Study the drawing (mm; zero at the part's minimum x, y, z) and answer. A direction names the side the tool comes from. Coordinates: 2 decimals unless noted, no trailing zeros. Order: outer loops, then holes, each group sorted by start corner. A loop starts at its lowest first (then second) coordinate and runs counter-clockwise, first axis right, second up. Notation, with made-up numbers: M 82.25,1.25 L 128.25,1.25 A22 cw 128.25,25.25 Z; hole C 7,59 d1. An arc over 180 degrees is marked long. Put each result on its own line as item: value.
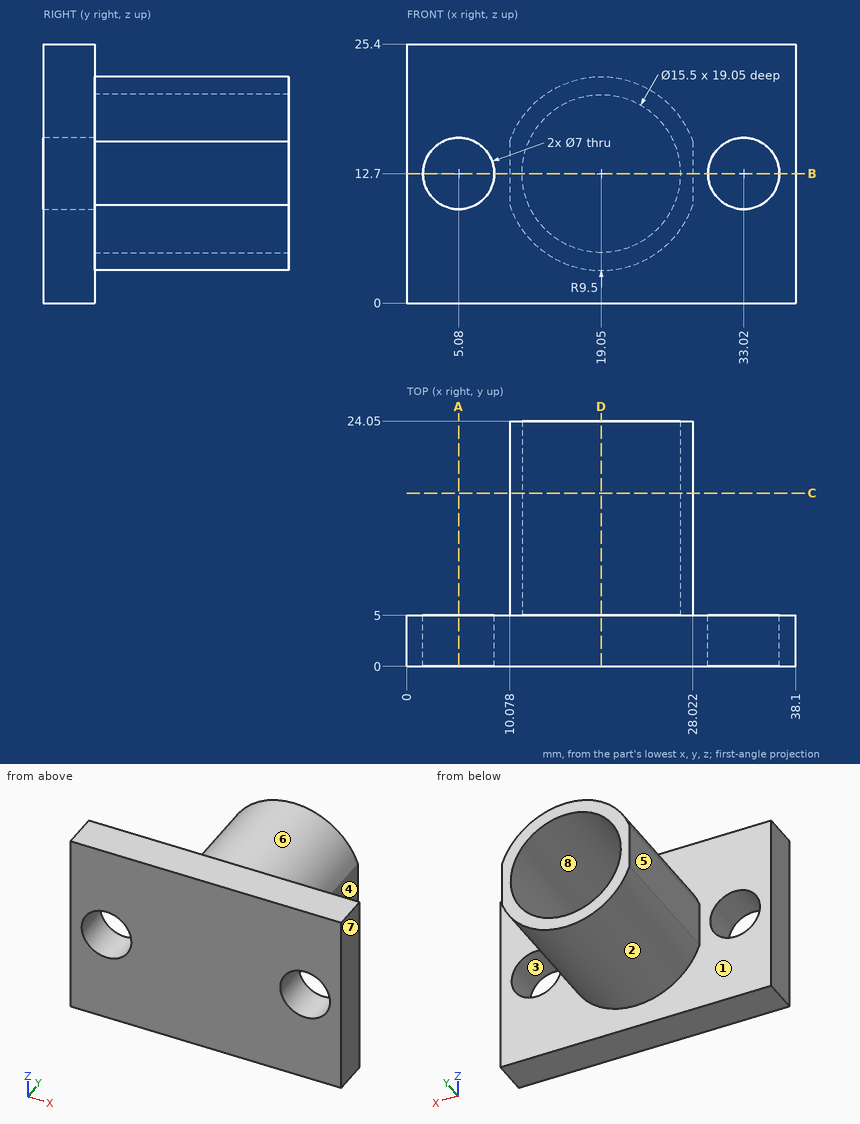
Q1. Find section D-D on x = 19.05. Write down the section's boundary in (y, z), plus the area to 3 significant figures.
Answers below:
outline: M 0,0 L 5,0 L 5,3.2 L 24.05,3.2 L 24.05,4.95 L 5,4.95 L 5,20.45 L 24.05,20.45 L 24.05,22.2 L 5,22.2 L 5,25.4 L 0,25.4 Z
area: 194 mm^2
Q2. Find section B-B on z = 12.7. Write down the section's boundary in (x, y).
Answers below:
outline: M 0,0 L 1.58,0 L 1.58,5 L 0,5 Z; M 8.58,0 L 29.52,0 L 29.52,5 L 28.02,5 L 28.02,24.05 L 26.8,24.05 L 26.8,5 L 11.3,5 L 11.3,24.05 L 10.08,24.05 L 10.08,5 L 8.58,5 Z; M 36.52,0 L 38.1,0 L 38.1,5 L 36.52,5 Z
Q3. Given pin 1 (4 mm diameter, centred on x = 14.5, z = 22, fed in from -Y); pin 2 (1.9 mm diameter, centred on y = 16, z = 14, fed in from +X); pin 3 (7 mm diameter, centred on y = 19, z = 14, fed in from -X); pin 4 (1.5 mm diameter, centred on x = 18.5, z = 15.5, fed in from +Y), each flat-ended and moving along its own axis, determine where each tip first touches the part or whether it passes through.
Answers below:
pin 1: stops at y = 0
pin 2: stops at x = 28.02
pin 3: stops at x = 10.08
pin 4: stops at y = 5
Q4. Find section A-A on x = 5.08. Write down the section's boundary in (y, z).
Answers below:
outline: M 0,0 L 5,0 L 5,9.2 L 0,9.2 Z; M 0,16.2 L 5,16.2 L 5,25.4 L 0,25.4 Z
Q5. For a pull along X with two mould halves and no side action, classify the marked faces 1, 2 and 3 as +X half, -X half, draft (parallel to the pull), parting line (faces both ways), or undercut.
Answers below:
face 1: draft
face 2: parting line
face 3: undercut
Q6. Consider line 1 along X through (y, z) = (2, 12.7); line 2 along X through (y, z) = (14.75, 12.7); line 3 along Y through (x, z) = (3, 21.25). Determine where each line is inside the solid, lowest interval first.
Answers below:
line 1: x = 0 to 1.58, 8.58 to 29.52, 36.52 to 38.1
line 2: x = 10.08 to 11.3, 26.8 to 28.02
line 3: y = 0 to 5
Q7. Find section C-C on y = 17. Write down the section's boundary in (x, z).
Answers below:
outline: M 10.08,9.58 A9.5 ccw 28.02,9.58 L 28.02,15.82 A9.5 ccw 10.08,15.82 Z; hole C 19.05,12.7 d15.5
Q8. A tool of negligible diameter and unlimited length cuts with its end or side. For the marked faces 4, 5, 6, 7 and 8, from which of +Z, -Z, +X, -X, +Y, -Y can it reach the whole face along a straight path? Write none if from no direction.
Answers below:
face 4: +Z, -Z, +X, +Y
face 5: +Z, -Z, -X, +Y
face 6: +Z, +Y
face 7: +Z, -Z, +X, +Y, -Y
face 8: +Y
